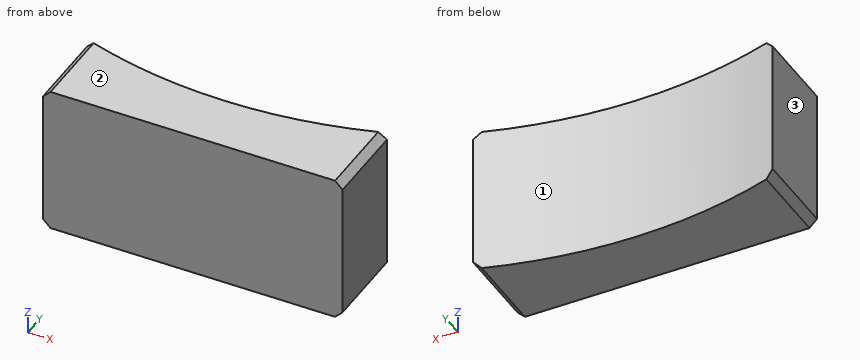
from build123d import *

# Parameters (mm, degrees)
BOSS_EXTRUDE1_DEPTH = 12.7
CHAMFER1_SIZE       = 0.635


with BuildPart() as part:
    # Sketch1 → Boss-Extrude1 (new body)
    with BuildSketch(Plane.XY):
        with BuildLine():
            Line((-12.7, 7.170396709), (-12.7, 0))
            Line((-12.7, 0), (12.7, 0))
            Line((12.7, 0), (12.7, 7.170396709))
            ThreePointArc((12.7, 7.170396709), (0, 5.08), (-12.7, 7.170396709))
        make_face()
    extrude(amount=BOSS_EXTRUDE1_DEPTH)

    # Chamfer1
    chamfer1_edges = [part.edges().sort_by_distance(p)[0] for p in [
        (12.7, 3.585198355, 12.7),
        (12.7, 3.585198355, 0),
        (-12.7, 3.585198355, 0),
        (-12.7, 3.585198355, 12.7),
    ]]
    chamfer(chamfer1_edges, length=CHAMFER1_SIZE)


solid = part.part
Here's how the part is built. I have some questions about the finished solid (model axes, mm). Face numbers are marked on the shaded views. Coordinates: 2 decimals unless noted, no trailing zeros. Order: outer loops, then holes, each group sorted by start corner. A loop starts at its lowest first (then second) coordinate and runs counter-clockwise, first axis right, second up. Notation, with made-up numbers: M -19,-28.75 L -5,-28.75 A17 ccw -5,1.25 Z; hole C 3,29 d7. An arc over 180 degrees is marked long. Answer as CSV lines item,"result". Start each with the question number.
1. For pin 1 (6 mm diameter, centred on x = -0.5, z = 10.5, fed in from +Y), with a flat end and sliding along its axis, tell me the tip position at first contact or that it passes through.
2. I need wall thicknesses on line 1 (Y direction, x = 9, z = 7.75); line 2 (Y direction, x = -6.5, z = 3.25). Which ranges of each line are inside material? Lowest first, please. Write a range as [from, to].
3. I want a section at B-B, the plane x = 1.25. Write out the boundary of the cut face in (y, z), and give its area (3 significant figures).
4. I want a section at A-A, the plane z = 5.75. Write out the boundary of the cut face in (x, y), and give its area (3 significant figures).
5. We'd pull the mould along X, two halves only. Please class the marked faces 1, 2 and 3: released by +X, released by -X, zero draft, split by the parting line, or undercut.
Recorded:
1,pin 1,"stops at y = 5.23"
2,line 1,"y = [0, 6.12]"
2,line 2,"y = [0, 5.62]"
3,outline,"M 0,0 L 5.1,0 L 5.1,12.7 L 0,12.7 Z"
3,area,"64.8 mm2"
4,outline,"M -12.7,0 L 12.7,0 L 12.7,7.17 A39.62 cw -12.7,7.17 Z"
4,area,"147 mm2"
5,face 1,"undercut"
5,face 2,"zero draft"
5,face 3,"released by -X"
